Study the drawing (mm; zero at the part's minimum x, y, z) and answer. A direction names the side the tool comes from. Round coordinates to 2 decimals unless told otherwise and drop trailing zeros. Write each loop counter-clockwise with the first axis right and the second up, starting at its lowest first coordinate (ties: lowest second). Pieces come first, ordered by that corner, then holes. Notation, with made-up numbers: M 49.25,59.25 L 81.25,59.25 A21 cw 81.25,75.25 Z; hole C 10,-19 d6. An arc over 180 degrees is marked long. Write each question's results on one line, items separated by ' | '.
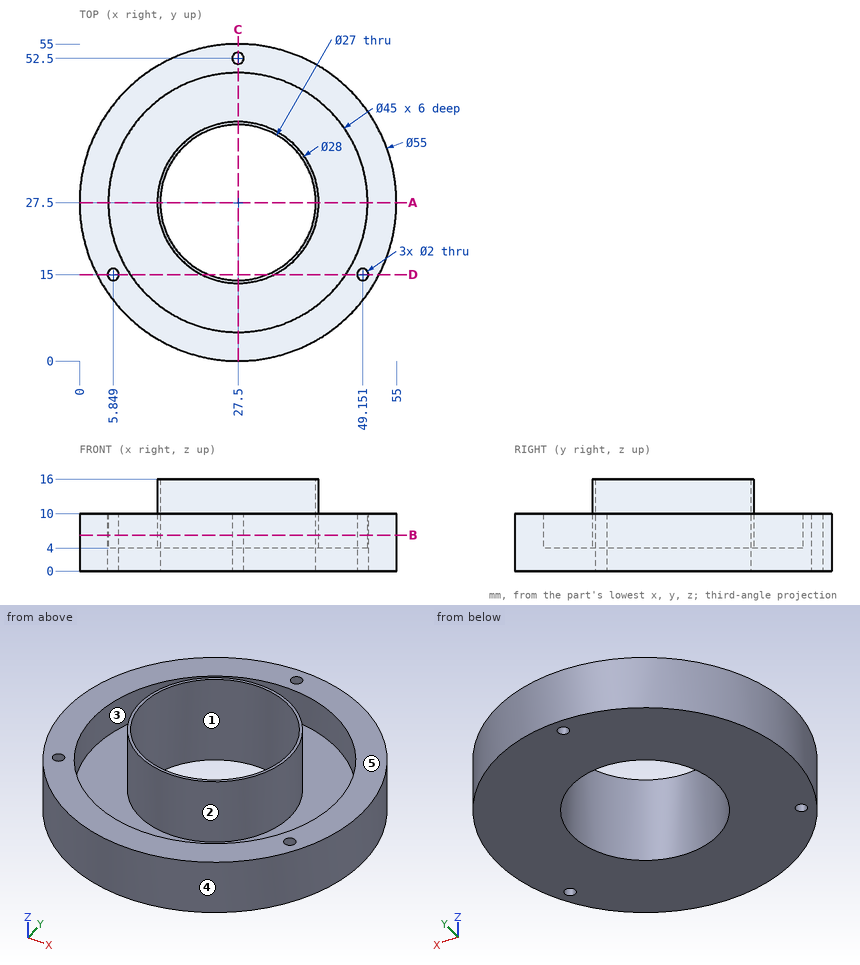
1) Section B-B (z = 6.25) is taken. Determine the outline of the cut face in (x, y).
Return value:
outline: C 27.5,27.5 d55; C 27.5,27.5 d28; hole C 5.85,15 d2; hole C 27.5,27.5 d45; hole C 27.5,27.5 d27; hole C 27.5,52.5 d2; hole C 49.15,15 d2
2) Find the intervals of material crossed by line 1 (Y direction, x = 27.5, z = 3.5); line 2 (Y direction, x = 27.5, z = 7.3); line 3 (Y direction, x = 16.5, z = 7) (1 decimal), in increasing order.
Return value:
line 1: 0 to 14, 41 to 51.5, 53.5 to 55 | line 2: 0 to 5, 13.5 to 14, 41 to 41.5, 50 to 51.5, 53.5 to 55 | line 3: 2.3 to 7.9, 18.8 to 19.7, 35.3 to 36.2, 47.1 to 52.7
3) Each of these flat-tipped pins is pushed along its axis until it touches: pin 1 (6 mm diameter, centred on y = 13.5, z = 4, fed in from +X) (1 decimal); pin 2 (4 mm diameter, centred on x = 44.5, z = 7, fed in from -Y). Where does it stop, or does it pass through?
Return value:
pin 1: x = 52.7 | pin 2: y = 4.45
4) A tool of negligible diameter and unlimited length cuts with its end or side. For the marked faces 1 and 2, from which of +Z, -Z, +X, -X, +Y, -Y can it reach the whole face along a straight path? Write none if from no direction.
Return value:
face 1: +Z, -Z | face 2: +Z
5) The mould has two halves that part along X. Classify the marked faces 3, 4 and 5: +X half, -X half, draft (parallel to the pull), parting line (faces both ways), or undercut.
Return value:
face 3: undercut | face 4: parting line | face 5: draft
6) Section A-A (y = 27.5) is taken. Determine the outline of the cut face in (x, z).
Return value:
outline: M 0,0 L 14,0 L 14,16 L 13.5,16 L 13.5,4 L 5,4 L 5,10 L 0,10 Z; M 41,0 L 55,0 L 55,10 L 50,10 L 50,4 L 41.5,4 L 41.5,16 L 41,16 Z
7) Section C-C (x = 27.5) is taken. Determine the outline of the cut face in (y, z), then the cut area to 3 significant figures.
Return value:
outline: M 0,0 L 14,0 L 14,16 L 13.5,16 L 13.5,4 L 5,4 L 5,10 L 0,10 Z; M 41,0 L 51.5,0 L 51.5,10 L 50,10 L 50,4 L 41.5,4 L 41.5,16 L 41,16 Z; M 53.5,0 L 55,0 L 55,10 L 53.5,10 Z | area: 164 mm²
8) Section D-D (y = 15) is taken. State how many separate pieces and enclosed holes the cut face has.
Return value:
separate pieces: 4 | enclosed holes: 0
